Could you check a few things on this model? Use its own coordinates, in mm. Face numbers are marked on the shaded views. Coordinates: 2 decimals unless noted, no trailing zeros. Write each loop counter-clockwise with the first axis right and the second up, starting at its lowest first coordinate (ties: lowest second). Pieces come first, ordered by that corner, then holes.
```python
from build123d import *

# Parameters (mm, degrees)
SKETCH1_R                    = 2.4892
SKETCH1_R_2                  = 1.5875
BASE_FLANGE1_DEPTH           = 2.286
EDGE_FLANGE2_DEPTH           = 169.545
EDGE_FLANGE3_STRIP_W         = 21.43
EDGE_FLANGE3_STRIP_H         = 2.286
EDGE_FLANGE3_STRIP_CUT_DEPTH = 169.545
EDGE_FLANGE3_DEPTH           = 169.545
EDGE_FLANGE3_PROFILE_W       = 169.545
EDGE_FLANGE3_PROFILE_H       = 25.781
EDGE_FLANGE3_PROFILE_R       = 1.5875
EDGE_FLANGE3_FLAT_DEPTH      = 2.286
EDGE_FLANGE6_DEPTH           = 151.257
EDGE_FLANGE7_STRIP_W         = 21.43
EDGE_FLANGE7_STRIP_H         = 2.286
EDGE_FLANGE7_STRIP_CUT_DEPTH = 151.257
EDGE_FLANGE7_DEPTH           = 151.257
EDGE_FLANGE7_PROFILE_W       = 151.257
EDGE_FLANGE7_PROFILE_H       = 13.23975
EDGE_FLANGE7_PROFILE_R       = 1.63195
EDGE_FLANGE7_FLAT_DEPTH      = 2.286
EDGE_FLANGE8_DEPTH           = 220.98
EDGE_FLANGE8_START           = -2.286
EDGE_FLANGE8_PROFILE_W       = 220.98
EDGE_FLANGE8_PROFILE_H       = 9.271
EDGE_FLANGE8_PROFILE_R       = 1.5875
EDGE_FLANGE8_FLAT_DEPTH      = 2.286
FILLET1_R                    = 2.54
FILLET2_R                    = 12.7
SKETCH35_W                   = 16.66875
SKETCH35_H                   = 152.4
SKETCH35_W_2                 = 38.1
SKETCH35_H_2                 = 3.429
CUT_EXTRUDE1_DEPTH           = 307.869010961
BOSS_EXTRUDE1_START          = -2.286
BOSS_EXTRUDE1_DEPTH          = 2.286
EDGE_FLANGE9_STRIP_W         = 21.43
EDGE_FLANGE9_STRIP_H         = 2.286
EDGE_FLANGE9_STRIP_CUT_DEPTH = 38.1
EDGE_FLANGE9_DEPTH           = 38.1
BOSS_EXTRUDE2_DEPTH          = 2.286
F_10_CLEARANCE_HOLE1_D       = 4.9784
FILLET3_R                    = 2.54
SKETCH43_R                   = 14.2875
CUT_EXTRUDE2_DEPTH           = 2.54


# Sheet-metal steps are written as plain solids
with BuildPart() as part:
    # Sketch1 → Base-Flange1 (new body)
    with BuildSketch(Plane.XY):
        Polygon((0, 0), (0, 171.45), (220.98, 171.45), (220.98, -21.59), (246.38, -21.59), (246.38, -72.39), (200.152, -72.39), (200.152, -18.415), (195.58, -18.415), (195.58, 152.4), (7.62, 152.4), (7.62, 0), align=None)
        with Locations((233.68, -59.69)):
            Circle(SKETCH1_R, mode=Mode.SUBTRACT)
        with Locations((212.852, -59.69)):
            Circle(SKETCH1_R, mode=Mode.SUBTRACT)
        with Locations((212.852, -34.29)):
            Circle(SKETCH1_R, mode=Mode.SUBTRACT)
        with Locations((233.68, -34.29)):
            Circle(SKETCH1_R, mode=Mode.SUBTRACT)
        with Locations((208.28, 117.7925)):
            Circle(SKETCH1_R, mode=Mode.SUBTRACT)
        with Locations((208.28, 92.3925)):
            Circle(SKETCH1_R, mode=Mode.SUBTRACT)
        with Locations((208.28, 66.9925)):
            Circle(SKETCH1_R, mode=Mode.SUBTRACT)
        with Locations((208.28, 41.5925)):
            Circle(SKETCH1_R, mode=Mode.SUBTRACT)
        with Locations((208.28, 16.1925)):
            Circle(SKETCH1_R, mode=Mode.SUBTRACT)
        with Locations((19.05, 161.925)):
            Circle(SKETCH1_R_2, mode=Mode.SUBTRACT)
        with Locations((55.626, 161.925)):
            Circle(SKETCH1_R_2, mode=Mode.SUBTRACT)
        with Locations((92.202, 161.925)):
            Circle(SKETCH1_R_2, mode=Mode.SUBTRACT)
        with Locations((128.778, 161.925)):
            Circle(SKETCH1_R_2, mode=Mode.SUBTRACT)
        with Locations((165.354, 161.925)):
            Circle(SKETCH1_R_2, mode=Mode.SUBTRACT)
        with Locations((201.93, 161.925)):
            Circle(SKETCH1_R_2, mode=Mode.SUBTRACT)
    extrude(amount=-BASE_FLANGE1_DEPTH)

    # Edge-Flange2 section (across the edge) → Edge-Flange2 (add)
    with BuildSketch(Plane(origin=(194.056, -18.415, -2.286), x_dir=(1, 0, 0), z_dir=(0, 1, 0))):
        with BuildLine():
            Line((-2.286, 1.143), (-2.286, 50.9905))
            Line((-2.286, 50.9905), (0, 50.9905))
            Line((0, 50.9905), (0, 1.143))
            ThreePointArc((0, 1.143), (0.334776949, 0.334776949), (1.143, 0))
            Line((1.143, 0), (1.524, 0))
            Line((1.524, 0), (1.524, -2.286))
            Line((1.524, -2.286), (1.143, -2.286))
            ThreePointArc((1.143, -2.286), (-1.281669153, -1.281669153), (-2.286, 1.143))
        make_face()
    extrude(amount=EDGE_FLANGE2_DEPTH)

    # Edge-Flange3 strip (across the edge) → Edge-Flange3 strip cut (cut)
    with BuildSketch(Plane(origin=(194.056, -18.415, -53.2765), x_dir=(0, 0, 1), z_dir=(0, 1, 0))):
        with Locations((-7.286, -1.143)):
            Rectangle(EDGE_FLANGE3_STRIP_W, EDGE_FLANGE3_STRIP_H)
    extrude(amount=EDGE_FLANGE3_STRIP_CUT_DEPTH, mode=Mode.SUBTRACT)

    # Edge-Flange3 bend section (across the edge) → Edge-Flange3 (add)
    with BuildSketch(Plane(origin=(194.056, -18.415, -53.2765), x_dir=(0, 0, 1), z_dir=(0, 1, 0))):
        with BuildLine():
            Line((0, 1.143), (2.286, 1.143))
            ThreePointArc((2.286, 1.143), (2.620776949, 0.334776949), (3.429, 0))
            Line((3.429, 0), (3.429, -2.286))
            ThreePointArc((3.429, -2.286), (1.004330847, -1.281669153), (0, 1.143))
        make_face()
    extrude(amount=EDGE_FLANGE3_DEPTH)

    # Edge-Flange3 profile (on flange) → Edge-Flange3 flat (add)
    with BuildSketch(Plane(origin=(194.056, 0, -53.2765), x_dir=(0, 1, 0), z_dir=(0, 0, -1))):
        with Locations((66.3575, 14.0335)):
            Rectangle(EDGE_FLANGE3_PROFILE_W, EDGE_FLANGE3_PROFILE_H)
        with Locations((139.7, 13.462)):
            Circle(EDGE_FLANGE3_PROFILE_R, mode=Mode.SUBTRACT)
        with Locations((115.464166667, 13.462)):
            Circle(EDGE_FLANGE3_PROFILE_R, mode=Mode.SUBTRACT)
        with Locations((91.228333333, 13.462)):
            Circle(EDGE_FLANGE3_PROFILE_R, mode=Mode.SUBTRACT)
        with Locations((66.9925, 13.462)):
            Circle(EDGE_FLANGE3_PROFILE_R, mode=Mode.SUBTRACT)
        with Locations((42.756666667, 13.462)):
            Circle(EDGE_FLANGE3_PROFILE_R, mode=Mode.SUBTRACT)
        with Locations((18.520833333, 13.462)):
            Circle(EDGE_FLANGE3_PROFILE_R, mode=Mode.SUBTRACT)
        with Locations((-5.715, 13.462)):
            Circle(EDGE_FLANGE3_PROFILE_R, mode=Mode.SUBTRACT)
    extrude(amount=-EDGE_FLANGE3_FLAT_DEPTH)

    # Edge-Flange6 section (across the edge) → Edge-Flange6 (add)
    with BuildSketch(Plane(origin=(9.144, 151.257, -2.286), x_dir=(-1, 0, 0), z_dir=(0, -1, 0))):
        with BuildLine():
            Line((-2.286, 1.143), (-2.286, 48.514))
            Line((-2.286, 48.514), (0, 48.514))
            Line((0, 48.514), (0, 1.143))
            ThreePointArc((0, 1.143), (0.334776949, 0.334776949), (1.143, 0))
            Line((1.143, 0), (1.524, 0))
            Line((1.524, 0), (1.524, -2.286))
            Line((1.524, -2.286), (1.143, -2.286))
            ThreePointArc((1.143, -2.286), (-1.281669153, -1.281669153), (-2.286, 1.143))
        make_face()
    extrude(amount=EDGE_FLANGE6_DEPTH)

    # Edge-Flange7 strip (across the edge) → Edge-Flange7 strip cut (cut)
    with BuildSketch(Plane(origin=(9.144, 151.257, -50.8), x_dir=(0, 0, 1), z_dir=(0, -1, 0))):
        with Locations((-7.286, -1.143)):
            Rectangle(EDGE_FLANGE7_STRIP_W, EDGE_FLANGE7_STRIP_H)
    extrude(amount=EDGE_FLANGE7_STRIP_CUT_DEPTH, mode=Mode.SUBTRACT)

    # Edge-Flange7 bend section (across the edge) → Edge-Flange7 (add)
    with BuildSketch(Plane(origin=(9.144, 151.257, -50.8), x_dir=(0, 0, 1), z_dir=(0, -1, 0))):
        with BuildLine():
            Line((0, 1.143), (2.286, 1.143))
            ThreePointArc((2.286, 1.143), (2.620776949, 0.334776949), (3.429, 0))
            Line((3.429, 0), (3.429, -2.286))
            ThreePointArc((3.429, -2.286), (1.004330847, -1.281669153), (0, 1.143))
        make_face()
    extrude(amount=EDGE_FLANGE7_DEPTH)

    # Edge-Flange7 profile (on flange) → Edge-Flange7 flat (add)
    with BuildSketch(Plane(origin=(9.144, 0, -50.8), x_dir=(0, 1, 0), z_dir=(0, 0, 1))):
        with Locations((75.6285, 7.762875)):
            Rectangle(EDGE_FLANGE7_PROFILE_W, EDGE_FLANGE7_PROFILE_H)
        with Locations((126.746, 7.14375)):
            Circle(EDGE_FLANGE7_PROFILE_R, mode=Mode.SUBTRACT)
        with Locations((83.08975, 7.14375)):
            Circle(EDGE_FLANGE7_PROFILE_R, mode=Mode.SUBTRACT)
        with Locations((39.4335, 7.14375)):
            Circle(EDGE_FLANGE7_PROFILE_R, mode=Mode.SUBTRACT)
    extrude(amount=EDGE_FLANGE7_FLAT_DEPTH)

    # Edge-Flange8 bend section (across the edge) → Edge-Flange8 (add)
    with BuildSketch(Plane(origin=(0, 172.72, -2.286), x_dir=(0, -1, 0), z_dir=(1, 0, 0))):
        with BuildLine():
            Line((-2.286, 1.143), (0, 1.143))
            ThreePointArc((0, 1.143), (0.334776949, 0.334776949), (1.143, 0))
            Line((1.143, 0), (1.27, 0))
            Line((1.27, 0), (1.27, -2.286))
            Line((1.27, -2.286), (1.143, -2.286))
            ThreePointArc((1.143, -2.286), (-1.281669153, -1.281669153), (-2.286, 1.143))
        make_face()
    extrude(amount=EDGE_FLANGE8_DEPTH)

    # Edge-Flange8 profile (on flange) → Edge-Flange8 flat (add)
    with BuildSketch(Plane(origin=(0, 172.72, -2.286), x_dir=(-1, 0, 0), z_dir=(0, -1, 0)).offset(EDGE_FLANGE8_START)):
        with Locations((-110.49, 5.7785)):
            Rectangle(EDGE_FLANGE8_PROFILE_W, EDGE_FLANGE8_PROFILE_H)
        with Locations((-12.7, 5.207)):
            Circle(EDGE_FLANGE8_PROFILE_R, mode=Mode.SUBTRACT)
        with Locations((-45.296666667, 5.207)):
            Circle(EDGE_FLANGE8_PROFILE_R, mode=Mode.SUBTRACT)
        with Locations((-77.893333333, 5.207)):
            Circle(EDGE_FLANGE8_PROFILE_R, mode=Mode.SUBTRACT)
        with Locations((-110.49, 5.207)):
            Circle(EDGE_FLANGE8_PROFILE_R, mode=Mode.SUBTRACT)
        with Locations((-143.086666667, 5.207)):
            Circle(EDGE_FLANGE8_PROFILE_R, mode=Mode.SUBTRACT)
        with Locations((-175.683333333, 5.207)):
            Circle(EDGE_FLANGE8_PROFILE_R, mode=Mode.SUBTRACT)
        with Locations((-208.28, 5.207)):
            Circle(EDGE_FLANGE8_PROFILE_R, mode=Mode.SUBTRACT)
    extrude(amount=EDGE_FLANGE8_FLAT_DEPTH)

    # Fillet1
    fillet1_edges = [part.edges().sort_by_distance(p)[0] for p in [
        (220.98, -18.415, -52.1335),
        (220.98, 151.13, -52.1335),
        (246.38, -21.59, -1.143),
        (200.152, -18.415, -1.143),
        (0, 173.863, -12.7),
        (220.98, 173.863, -12.7),
    ]]
    fillet(fillet1_edges, radius=FILLET1_R)

    # Fillet2
    fillet2_edges = [part.edges().sort_by_distance(p)[0] for p in [
        (220.98, -21.59, -1.143),
    ]]
    fillet(fillet2_edges, radius=FILLET2_R)

    # Sketch35 → Cut-Extrude1 (cut, through all)
    with BuildSketch(Plane.XY):
        with Locations((3.095625, 76.2)):
            Rectangle(SKETCH35_W, SKETCH35_H)
        with Locations((19.05, 173.2915)):
            Rectangle(SKETCH35_W_2, SKETCH35_H_2)
    extrude(amount=-CUT_EXTRUDE1_DEPTH, mode=Mode.SUBTRACT)

    # Sketch36 → Boss-Extrude1 (add)
    with BuildSketch(Plane.XY.offset(BOSS_EXTRUDE1_START)):
        with BuildLine():
            Line((36.83, 171.577), (0, 171.577))
            Line((0, 171.577), (0, 190.5))
            Line((0, 190.5), (27.305, 190.5))
            Line((27.305, 190.5), (27.305, 181.102))
            ThreePointArc((27.305, 181.102), (30.094807909, 174.366807909), (36.83, 171.577))
        make_face()
    extrude(amount=BOSS_EXTRUDE1_DEPTH)

    # Edge-Flange9 strip (across the edge) → Edge-Flange9 strip cut (cut)
    with BuildSketch(Plane.XZ.offset(-190.5)):
        with Locations((-7.286, -1.143)):
            Rectangle(EDGE_FLANGE9_STRIP_W, EDGE_FLANGE9_STRIP_H)
    extrude(amount=EDGE_FLANGE9_STRIP_CUT_DEPTH, mode=Mode.SUBTRACT)

    # Edge-Flange9 section (across the edge) → Edge-Flange9 (add)
    with BuildSketch(Plane.XZ.offset(-190.5)):
        with BuildLine():
            Line((0, 1.143), (0, 12.954))
            Line((0, 12.954), (2.286, 12.954))
            Line((2.286, 12.954), (2.286, 1.143))
            ThreePointArc((2.286, 1.143), (2.620776949, 0.334776949), (3.429, 0))
            Line((3.429, 0), (3.429, -2.286))
            ThreePointArc((3.429, -2.286), (1.004330847, -1.281669153), (0, 1.143))
        make_face()
    extrude(amount=EDGE_FLANGE9_DEPTH)

    # Sketch40 → Boss-Extrude2 (add)
    with BuildSketch(Plane(origin=(2.286, 0, 0), x_dir=(0, 0, -1), z_dir=(1, 0, 0))):
        Polygon((-12.954, 190.5), (-12.954, 203.2), (2.286, 203.2), (2.286, 191.77), (-1.143, 191.77), (-1.143, 190.5), align=None)
        Polygon((-12.954, 152.4), (-12.954, 139.7), (2.286, 139.7), (2.286, 151.13), (-1.143, 151.13), (-1.143, 152.4), align=None)
    extrude(amount=-BOSS_EXTRUDE2_DEPTH)

    # #10 Clearance Hole1 (through all)
    with Locations(Plane(origin=(2.286, 0, 0), x_dir=(0, 0, -1), z_dir=(1, 0, 0))):
        with Locations((-4.66725, 196.9643), (-4.66725, 147.0914)):
            Hole(F_10_CLEARANCE_HOLE1_D / 2)

    # Fillet3
    fillet3_edges = [part.edges().sort_by_distance(p)[0] for p in [
        (27.305, 190.5, -1.143),
        (1.143, 203.2, 12.954),
        (1.143, 203.2, -2.286),
        (1.143, 139.7, -2.286),
        (1.143, 139.7, 12.954),
    ]]
    fillet(fillet3_edges, radius=FILLET3_R)

    # Sketch43 → Cut-Extrude2 (cut)
    with BuildSketch(Plane.ZY.offset(-191.77)):
        with Locations((-26.63825, 6.9215)):
            Circle(SKETCH43_R)
        with Locations((-26.63825, 46.5455)):
            Circle(SKETCH43_R)
        with Locations((-26.63825, 86.1695)):
            Circle(SKETCH43_R)
        with Locations((-26.63825, 125.7935)):
            Circle(SKETCH43_R)
    extrude(amount=-CUT_EXTRUDE2_DEPTH, mode=Mode.SUBTRACT)


solid = part.part
```
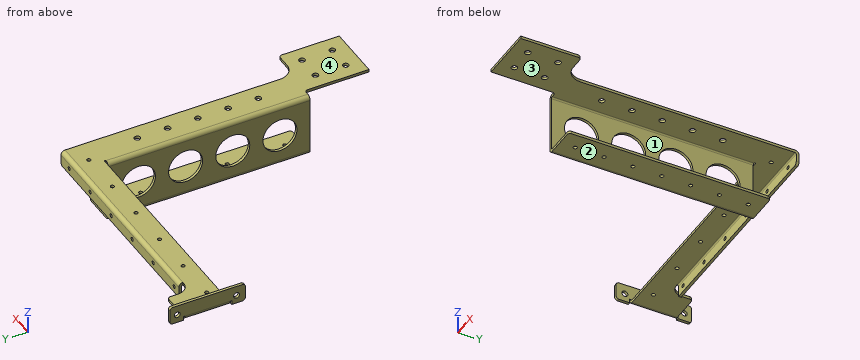
1. For pin 1 (5.5 mm diameter, centred on x = 233.68, y = -59.69, fed in from -Z); pin 2 (4 mm diameter, centred on y = 196.96, z = 4.67, fed in from -X); pin 3 (10 mm diameter, centred on x = 33.5, z = 0.5, fed in from -Y); pin 4 (11 mm diameter, centred on y = 99, z = -7, fed in from +X), each with a flat end and sliding along its axis, tell me the tip position at first contact or that it passes through.
Verdict:
pin 1: stops at z = -2.29
pin 2: passes through
pin 3: stops at y = 152.4
pin 4: stops at x = 220.98
2. Please list where these lines run through material, in increasing order: line 1 along X through (y, z) = (60, -17.5); line 2 along Z through (x, y) = (213.5, 59.5); line 3 along X through (y, z) = (168, 3).
Verdict:
line 1: x = 191.77 to 194.06
line 2: z = -53.28 to -50.99, -2.29 to 0
line 3: x = 0 to 2.29
3. I want a section at B-B on y = -48.5. Please give me the cut outline in (x, z).
Verdict:
outline: (200.15, -2.29) - (246.38, -2.29) - (246.38, 0) - (200.15, 0) - close
4. I want a section at A-A on z = -45. Please give me the cut outline in (x, y) (3 decimals), plus the area to 3 significant figures.
Verdict:
outline: (191.77, -18.415) - (194.056, -18.415) - (194.056, 151.13) - (191.77, 151.13) - close
area: 388 mm2
5. If we mould it in two halves opening along Z, with no side actions, what happens to the marked faces 1, 2, 3 and 4? For each: pulls with the +Z half, pulls with the -Z half, needs draft (parallel to the pull), parting line crosses it, or undercut.
Verdict:
face 1: undercut
face 2: pulls with the -Z half
face 3: undercut
face 4: pulls with the +Z half
